CAD build for the part. Positions are in the model's coordinates, mm. Coordinates: 2 decimals unless noted, no trailing zeros. Loops run counter-clockwise (first coordinate to the right, second up) from the corner with the lowest first, then second, coordinate; pieces in that order, holes last. Notation, with made-up numbers: (-39.5, 6) -> (-4.5, 6) arc R25 cw to (-4.5, 25) -> close; hole circle Ø2 at (52.5, 50.25). An arc over 180 degrees is marked (long way). Answer as a JSON object with one key per item and string values. Group by question number.
Autodesk Inventor part; units mm, degrees
ref_plane "YZ Plane" through (0, 0, 0) normal (1, 0, 0) x (0, 1, 0)
ref_plane "XZ Plane" through (0, 0, 0) normal (0, 1, 0) x (-1, 0, 0)
ref_plane "XY Plane" through (0, 0, 0) normal (0, 0, 1) x (1, 0, 0)
sketch "Sketch1" plane through (0, 0, 0) normal (0, 0, 1) x (1, 0, 0)
  line L0 (1.7529, 25) -> (4.7529, 25)
  line L1 (4.7529, 35) -> (1.7529, 35)
  line L2 (1.7529, 35) -> (1.7529, 25)
  line L3 (1.7529, -25) -> (4.7529, -25)
  line L4 (4.7529, -35) -> (1.7529, -35)
  line L5 (1.7529, -35) -> (1.7529, -25)
  line L6 (26.0029, -10.7424) -> (26.0029, 10.7264)
  line L7 (38.0029, -20.6235) -> (38.0029, -15.7736)
  line L8 (38.0029, 15.7576) -> (38.0029, 20.6075)
  line L9 (36.251, 13.773) -> (34.6269, 13.57)
  line L10 (29.6269, 12.945) -> (27.7548, 12.711)
  line L11 (36.251, -13.789) -> (34.6271, -13.586)
  line L12 (29.6269, -12.961) -> (27.7548, -12.727)
  arc A0 (26.0029, -10.7424) -> (27.7548, -12.727) centre (28.0029, -10.7424) ccw
  arc A1 (27.7548, 12.711) -> (26.0029, 10.7264) centre (28.0029, 10.7264) ccw
  arc A2 (38.0029, -15.7736) -> (36.251, -13.789) centre (36.0029, -15.7736) ccw
  arc A3 (36.251, 13.773) -> (38.0029, 15.7576) centre (36.0029, 15.7576) ccw
  arc A4 (30.5029, -13.9533) -> (29.6269, -12.961) centre (29.5029, -13.9533) ccw
  arc A5 (34.6271, -13.586) -> (33.5031, -14.5783) centre (34.5031, -14.5783) ccw
  arc A6 (33.5029, 14.5623) -> (34.6269, 13.57) centre (34.5029, 14.5623) ccw
  arc A7 (29.6269, 12.945) -> (30.5029, 13.9373) centre (29.5029, 13.9373) ccw
  arc A8 (38.0029, 20.6075) -> (37.7807, 21.5238) centre (36.0029, 20.6075) ccw
  arc A9 (37.7807, -21.5398) -> (38.0029, -20.6235) centre (36.0029, -20.6235) ccw
  line L13 (4.7529, -35) -> (4.7529, -44.9628)
  line L14 (4.7529, 35) -> (4.7529, 44.9468)
  line L15 (4.7529, 25) -> (4.7529, -25)
  line L16 (9.7529, -15.508) -> (19.7529, -15.508)
  line L17 (19.7529, -15.508) -> (19.7529, -12.508)
  line L18 (19.7529, -12.508) -> (9.7529, -12.508)
  line L19 (9.7529, -12.508) -> (9.7529, -15.508)
  line L20 (9.7529, 12.492) -> (19.7529, 12.492)
  line L21 (19.7529, 12.492) -> (19.7529, 15.492)
  line L22 (19.7529, 15.492) -> (9.7529, 15.492)
  line L23 (9.7529, 15.492) -> (9.7529, 12.492)
  arc A10 (4.7529, -44.9628) -> (5.9649, -45.9401) centre (5.7529, -44.9628) ccw
  arc A11 (5.9649, 45.9241) -> (4.7529, 44.9468) centre (5.7529, 44.9468) ccw
  line L24 (19.7529, -6.008) -> (11.7529, -6.008)
  line L25 (9.7529, -4.008) -> (9.7529, 3.992)
  line L26 (11.7529, 5.992) -> (19.7529, 5.992)
  line L27 (21.7529, 3.992) -> (21.7529, -4.008)
  line L28 (11.7529, 21.992) -> (19.7529, 21.992)
  line L29 (21.7529, 23.992) -> (21.7529, 31.992)
  line L30 (19.7529, 33.992) -> (11.7529, 33.992)
  line L31 (9.7529, 31.992) -> (9.7529, 23.992)
  line L32 (11.7529, -22.008) -> (19.7529, -22.008)
  line L33 (21.7529, -24.008) -> (21.7529, -32.008)
  line L34 (19.7529, -34.008) -> (11.7529, -34.008)
  line L35 (9.7529, -32.008) -> (9.7529, -24.008)
  arc A12 (11.7529, 5.992) -> (9.7529, 3.992) centre (11.7529, 3.992) ccw
  arc A13 (21.7529, 3.992) -> (19.7529, 5.992) centre (19.7529, 3.992) ccw
  arc A14 (19.7529, -6.008) -> (21.7529, -4.008) centre (19.7529, -4.008) ccw
  arc A15 (9.7529, -4.008) -> (11.7529, -6.008) centre (11.7529, -4.008) ccw
  arc A16 (11.7529, -22.008) -> (9.7529, -24.008) centre (11.7529, -24.008) ccw
  arc A17 (21.7529, -24.008) -> (19.7529, -22.008) centre (19.7529, -24.008) ccw
  arc A18 (19.7529, -34.008) -> (21.7529, -32.008) centre (19.7529, -32.008) ccw
  arc A19 (9.7529, -32.008) -> (11.7529, -34.008) centre (11.7529, -32.008) ccw
  arc A20 (11.7529, 33.992) -> (9.7529, 31.992) centre (11.7529, 31.992) ccw
  arc A21 (21.7529, 31.992) -> (19.7529, 33.992) centre (19.7529, 31.992) ccw
  arc A22 (19.7529, 21.992) -> (21.7529, 23.992) centre (19.7529, 23.992) ccw
  arc A23 (9.7529, 23.992) -> (11.7529, 21.992) centre (11.7529, 23.992) ccw
  line L36 (31.7529, 29.1156) -> (31.7529, 22.992)
  line L37 (30.7529, 21.992) -> (27.7529, 21.992)
  line L38 (26.7529, 22.992) -> (26.7529, 34.6104)
  arc A24 (37.7807, 21.5238) -> (32.6427, 29.4288) centre (-3.9971, -0.008) ccw
  arc A25 (26.0307, 36.149) -> (5.9649, 45.9241) centre (-3.9971, -0.008) ccw
  line L39 (27.7529, -22.008) -> (30.7529, -22.008)
  line L40 (31.7529, -23.008) -> (31.7529, -29.1317)
  line L41 (26.7529, -34.6265) -> (26.7529, -23.008)
  arc A26 (5.9649, -45.9401) -> (26.0307, -36.1651) centre (-3.9971, -0.008) ccw
  arc A27 (32.6427, -29.4448) -> (37.7807, -21.5398) centre (-3.9971, -0.008) ccw
  arc A28 (32.6427, 29.4288) -> (31.7529, 29.1156) centre (32.2529, 29.1156) ccw
  arc A29 (31.7529, -29.1317) -> (32.6427, -29.4448) centre (32.2529, -29.1317) ccw
  arc A30 (26.0307, -36.1651) -> (26.7529, -34.6265) centre (24.7529, -34.6265) ccw
  arc A31 (26.7529, 34.6104) -> (26.0307, 36.149) centre (24.7529, 34.6104) ccw
  arc A32 (30.7529, 21.992) -> (31.7529, 22.992) centre (30.7529, 22.992) ccw
  arc A33 (26.7529, 22.992) -> (27.7529, 21.992) centre (27.7529, 22.992) ccw
  arc A34 (31.7529, -23.008) -> (30.7529, -22.008) centre (30.7529, -23.008) ccw
  arc A35 (27.7529, -22.008) -> (26.7529, -23.008) centre (27.7529, -23.008) ccw
  arc A36 (30.5029, -17.9841) -> (33.5031, -18.008) centre (32.0029, -18.008) ccw
  arc A37 (33.5029, 17.992) -> (30.5029, 17.992) centre (32.0029, 17.992) ccw
  line L42 (30.5029, 17.992) -> (30.5029, 13.9373)
  line L43 (33.5029, 17.992) -> (33.5029, 14.5623)
  line L44 (30.5029, -18.032) -> (30.5029, -13.9533)
  line L45 (33.5031, -18.008) -> (33.5031, -14.5783)
  point P0 (4.7529, -46.1863)
  point P1 (4.7529, 46.1703)
  point P2 (38.0029, -21.103)
  point P3 (38.0029, 21.087)
  point P4 (38.0029, -14.008)
  point P5 (38.0029, 13.992)
  point P6 (26.0029, -12.508)
  point P7 (9.7529, 5.992)
  point P8 (9.7529, -6.008)
  point P9 (21.7529, 5.992)
  point P10 (21.7529, 33.992)
  point P11 (21.7529, 21.992)
  point P12 (9.7529, 33.992)
  point P13 (21.7529, -34.008)
  point P14 (21.7529, -22.008)
  point P15 (9.7529, -34.008)
  point P16 (26.7529, 35.5369)
  point P17 (31.7529, 30.5033)
  point P18 (26.7529, -22.008)
  point P19 (26.7529, -35.5529)
  point P20 (31.7529, -30.5193)
  dimension "d13" = 10
  dimension "d17" = 10
  dimension "d70" = 3
  dimension "d72" = 3
  dimension "d88" = 28
  dimension "d90" = 1.5
  dimension "d92" = 14
  dimension "d99" = 2
  dimension "d100" = 2
  dimension "d101" = 1
  dimension "d102" = 2
  dimension "d105" = 10
  dimension "d106" = 3
  dimension "d107" = 10
  dimension "d108" = 3
  dimension "d109" = 5
  dimension "d110" = 5
  dimension "d111" = 25
  dimension "d112" = 12.5
  dimension "d115" = 1
  dimension "d117" = 8.75
  dimension "d118" = 12
  dimension "d119" = 12
  dimension "d120" = 5
  dimension "d121" = 6.5
  dimension "d123" = 5
  dimension "d126" = 6.5
  dimension "d127" = 12
  dimension "d128" = 12
  dimension "d129" = 6.5
  dimension "d130" = 12
  dimension "d131" = 12
  dimension "d132" = 2
  dimension "d135" = 5
  dimension "d136" = 5
  dimension "d137" = 5
  dimension "d138" = 6.5
  dimension "d139" = 5
  dimension "d140" = 5
  dimension "d141" = 0.5
  dimension "d142" = 2
  dimension "d143" = 1
  dimension "d144" = 3
  dimension "d147" = 4
  dimension "d148" = 4
extrude "Extrusion8" add sketch "Sketch1" along normal blind 3
properties part number "OpenROV 2.3 Dev EBoard Plug Mount"
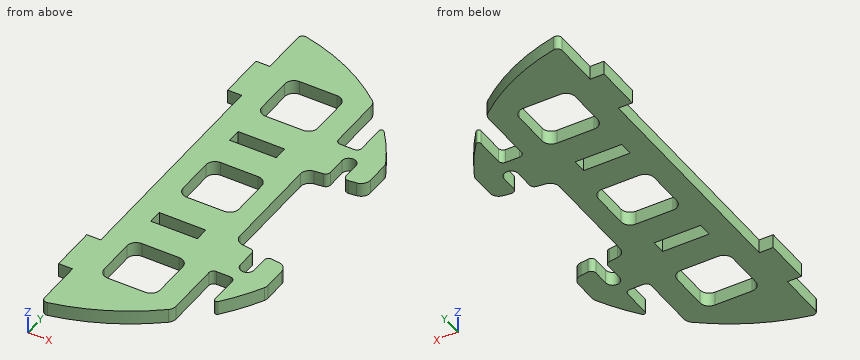
Item 1: Band-saw the part on D-D, the plane y = 3. List the corners of the cut face in (x, z).
Item 2: Band-saw the part on C-C, the plane z = 2.3. Count the separate pieces of the cut face and the enclosed holes in it, and give its area (3 significant figures).
Item 3: Drill centre lines: L1, parallel to X at y = 1.5, z = 1.05; L2, parallel to Y at x = 21, z = 2.75; L3, parallel to X at y = -32, z = 1.15. Where is each one in solid material? Low to high.
Item 4: Band-saw the part on B-B, the plane y = -26. List the corners of the cut face in (x, z).
Item 5: Band-saw the part on A-A, the plane y = 31. List the corners of the cut face in (x, z).
Item 6: Flat gauge pins, fed straight in: P1, Ø0.9, axis at y = 14, z = 1, coming from the -X side; P2, Ø0.9, axis at y = 2.5, z = 2, coming from the +X side; P3, Ø5, axis at x = 18, y = -2, coming from the +Z side; P4, Ø0.9, axis at x = 4, z = 1.5, coming from the +Y side. Where does each tip first touch, or does it go through?
Reply:
{
 "1": {"outline": "(4.75, 0) -> (9.75, 0) -> (9.75, 3) -> (4.75, 3) -> close; (21.75, 0) -> (26, 0) -> (26, 3) -> (21.75, 3) -> close"},
 "2": {"separate pieces": "1", "enclosed holes": "5", "area": "1,620 mm²"},
 "3": {"L1": "4.75 to 9.75, 21.75 to 26", "L2": "-39.81 to -33.57, -22.44 to -5.57, 5.56 to 22.43, 33.56 to 39.79", "L3": "1.75 to 9.75, 21.75 to 26.75"},
 "4": {"outline": "(1.75, 0) -> (9.75, 0) -> (9.75, 3) -> (1.75, 3) -> close; (21.75, 0) -> (26.75, 0) -> (26.75, 3) -> (21.75, 3) -> close; (31.75, 0) -> (35.16, 0) -> (35.16, 3) -> (31.75, 3) -> close"},
 "5": {"outline": "(1.75, 0) -> (9.75, 0) -> (9.75, 3) -> (1.75, 3) -> close; (21.75, 0) -> (26.75, 0) -> (26.75, 3) -> (21.75, 3) -> close"},
 "6": {"P1": "x = 4.75", "P2": "x = 26", "P3": "through", "P4": "y = 35"}
}
